Read the model definition and answer for the solid it produces. Units are mm, in the model's axes. Face numbers are marked on the shaded views. A direction names the side the tool comes from. Coordinates: 2 decimals unless noted, no trailing zeros. Write each loop counter-clockwise with the first axis right and the second up, starting at its lowest first coordinate (ties: lowest second). Pieces come first, ordered by that corner, then holes. Notation, with made-up numbers: (13.5, 28) -> (28.5, 28) arc R9 ccw to (28.5, 36) -> close; hole circle Ø4 at (15.25, 27). An arc over 180 degrees is marked (long way). Return JSON: item names as keys, results as strings.
from build123d import *

# Parameters (mm, degrees)
SKETCH1_W           = 50
SKETCH1_H           = 50
BOSS_EXTRUDE1_DEPTH = 41.25
SKETCH2_R           = 1.5
CUT_EXTRUDE1_DEPTH  = 6
SKETCH3_R           = 21
BOSS_EXTRUDE2_DEPTH = 26.5
FILLET1_R           = 3


with BuildPart() as part:
    # Sketch1 → Boss-Extrude1 (new body)
    with BuildSketch(Plane(origin=(0, 0, 0), x_dir=(1, 0, 0), z_dir=(0, 1, 0))):
        with Locations((25, 25)):
            Rectangle(SKETCH1_W, SKETCH1_H)
    extrude(amount=BOSS_EXTRUDE1_DEPTH)

    # Sketch2 → Cut-Extrude1 (cut)
    with BuildSketch(Plane.XZ):
        with Locations((5, -5)):
            Circle(SKETCH2_R)
        with Locations((45, -45)):
            Circle(SKETCH2_R)
    extrude(amount=-CUT_EXTRUDE1_DEPTH, mode=Mode.SUBTRACT)

    # Sketch3 → Boss-Extrude2 (add)
    with BuildSketch(Plane(origin=(0, 41.25, 0), x_dir=(1, 0, 0), z_dir=(0, 1, 0))):
        with Locations((25, 25)):
            Circle(SKETCH3_R)
    extrude(amount=BOSS_EXTRUDE2_DEPTH)

    # Fillet1
    fillet1_edges = [part.edges().sort_by_distance(p)[0] for p in [
        (4, 67.75, -25),
        (0, 20.625, 0),
        (50, 20.625, 0),
        (50, 20.625, -50),
        (0, 20.625, -50),
    ]]
    fillet(fillet1_edges, radius=FILLET1_R)


solid = part.part
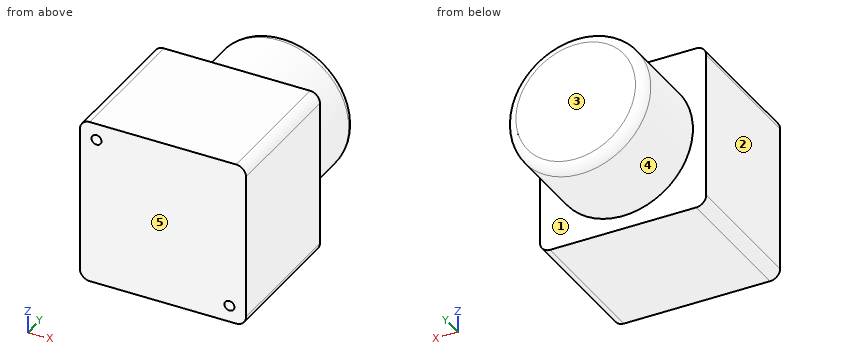
1. The part is cut by section B-B (x = 25). Determine the outline of the cut face in (y, z), then the cut area to 3 significant figures.
Taken from the geometry:
{"outline": "(0, -50) -> (41.25, -50) -> (41.25, -46) -> (64.75, -46) arc R3 ccw to (67.75, -43) -> (67.75, -7) arc R3 ccw to (64.75, -4) -> (41.25, -4) -> (41.25, 0) -> (0, 0) -> close", "area": "3,170 mm2"}
2. For a pull along Y with two mould halves and no side action, classify the marked faces 3, 4 and 5 as +Y half, -Y half, draft (parallel to the pull), parting line (faces both ways), or undercut.
Taken from the geometry:
{"face 3": "+Y half", "face 4": "draft", "face 5": "-Y half"}
3. The part is cut by section A-A (z = -25). Determine the outline of the cut face in (x, y), then the cut area to 3 significant figures.
Taken from the geometry:
{"outline": "(0, 0) -> (50, 0) -> (50, 41.25) -> (46, 41.25) -> (46, 64.75) arc R3 ccw to (43, 67.75) -> (7, 67.75) arc R3 ccw to (4, 64.75) -> (4, 41.25) -> (0, 41.25) -> close", "area": "3,170 mm2"}
4. Consider L1, parallel to Z at x = 5, y = 2; L2, parallel to Y at x = 47, z = -38; L3, parallel to Z at x = 45, y = 1.8. Determine where each line is inside the solid, lowest interval first.
Taken from the geometry:
{"L1": "z = -50 to -6.5, -3.5 to 0", "L2": "y = 0 to 41.25", "L3": "z = -50 to -46.5, -43.5 to 0"}
5. Flat-ended cylindrical pins translate along their axes: pin 1 Ø1.8 at (x, z) = (5, -5) entering from +Y; pin 2 Ø6 at (x, y) = (44, 52) entering from -Z; pin 3 Ø10 at (x, y) = (14, 50.5) entering from -Z. Find the tip coordinate at first contact, or state that the pin passes through.
Taken from the geometry:
{"pin 1": "stops at y = 41.25", "pin 2": "stops at z = -38.6", "pin 3": "stops at z = -45.12"}
6. A tool of negligible diameter and unlimited length cuts with its end or side. For the marked faces 1 and 2, from which of +Z, -Z, +X, -X, +Y, -Y can it reach the whole face along a straight path? Write none if from no direction.
Taken from the geometry:
{"face 1": "+Y", "face 2": "+Z, -Z, -X, +Y, -Y"}
7. The part is cut by section C-C (y = 46). Determine the outline of the cut face in (x, z).
Taken from the geometry:
{"outline": "circle Ø42 at (25, -25)"}
